from build123d import *

# Parameters (mm, degrees)
BOSS_EXTRUDE1_DEPTH      = 15.494
BOSS_EXTRUDE1_DEPTH_BACK = 15.494
SKETCH1_R                = 9.7409
SKETCH1_R_2              = 1.016
CHAMFER2_SIZE            = 4.7625
CHAMFER2_SIZE2           = 2.749630657
CHAMFER3_SIZE            = 4.7625
CHAMFER3_SIZE2           = 2.749630657


with BuildPart() as part:
    # Sketch1 → Boss-Extrude1 (new, two sides: drawn at the far end of the back side and taken through both)
    with BuildSketch(Plane.XY.offset(-BOSS_EXTRUDE1_DEPTH_BACK)):
        Circle(SKETCH1_R)
        Circle(SKETCH1_R_2, mode=Mode.SUBTRACT)
    extrude(amount=BOSS_EXTRUDE1_DEPTH + BOSS_EXTRUDE1_DEPTH_BACK)

    # Chamfer2
    chamfer2_edges = [part.edges().sort_by_distance(p)[0] for p in [
        (-9.7409, 0, -15.494),
    ]]
    chamfer2_side = [part.faces().sort_by_distance(p)[0] for p in [
        (-9.7409, 0, -7.747),
    ]]
    chamfer(chamfer2_edges, length=CHAMFER2_SIZE, length2=CHAMFER2_SIZE2, reference=chamfer2_side[0])

    # Chamfer3
    chamfer3_edges = [part.edges().sort_by_distance(p)[0] for p in [
        (-9.7409, 0, 15.494),
    ]]
    chamfer3_side = [part.faces().sort_by_distance(p)[0] for p in [
        (-9.7409, 0, 2.38125),
    ]]
    chamfer(chamfer3_edges, length=CHAMFER3_SIZE, length2=CHAMFER3_SIZE2, reference=chamfer3_side[0])


solid = part.part
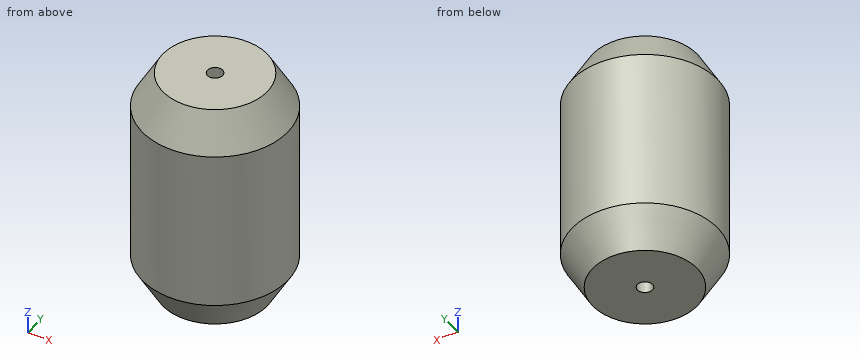
Could you check a few things on this model? Use its own coordinates, in mm. Give positions to 0.01 mm unless a question says otherwise; leave off trailing zeros. Write each loop counter-clockwise with the first axis right and the second up, starting at its lowest first coordinate (ties: lowest second). Pieces come first, ordered by that corner, then holes. Notation, with made-up numbers: (49.5, -8) -> (106.5, -8) arc R19 ccw to (106.5, 29) -> close; hole circle Ø11 at (31.25, -36.75). An arc over 180 degrees is marked (long way). Answer as a JSON object with one key per item and string values.
Q1. Suppose I cut it at D-D on z = 11.5. Write out the boundary of the cut face in (x, y), then the cut area to 3 significant figures.
Taken from the geometry:
{"outline": "circle Ø18.59 at (0, 0); hole circle Ø2.03 at (0, 0)", "area": "268 mm²"}
Q2. Suppose I cut it at A-A on x = 0. Write out the boundary of the cut face in (y, z), then the cut area to 3 significant figures.
Taken from the geometry:
{"outline": "(-9.74, -10.73) -> (-6.99, -15.49) -> (-1.02, -15.49) -> (-1.02, 15.49) -> (-6.99, 15.49) -> (-9.74, 10.73) -> close; (1.02, -15.49) -> (6.99, -15.49) -> (9.74, -10.73) -> (9.74, 10.73) -> (6.99, 15.49) -> (1.02, 15.49) -> close", "area": "515 mm²"}
Q3. Please list where these lines run through material, in increasing order: L1, parallel to Y at x = 0, z = -8; L2, parallel to X at y = -0.75, z = 2.5; L3, parallel to Y at x = -1.75, z = 8.
Taken from the geometry:
{"L1": "y = -9.74 to -1.02, 1.02 to 9.74", "L2": "x = -9.71 to -0.69, 0.69 to 9.71", "L3": "y = -9.58 to 9.58"}
Q4. Will these pins go through, and if not, where does the flat tip stop? pin 1 Ø6 at (y, z) = (-5, 7) entering from +X; pin 2 Ø1 at (y, z) = (-7.5, -9) entering from -X; pin 3 Ø1.2 at (x, y) = (0, 0) entering from -Z; pin 4 Ø2 at (x, z) = (-2, 3.5) entering from +Y.
Taken from the geometry:
{"pin 1": "stops at x = 9.53", "pin 2": "stops at x = -6.77", "pin 3": "passes through", "pin 4": "stops at y = 9.69"}
Q5. Suppose I cut it at C-C on z = -4.5. Write out the boundary of the cut face in (x, y), then the cut area to 3 significant figures.
Taken from the geometry:
{"outline": "circle Ø19.48 at (0, 0); hole circle Ø2.03 at (0, 0)", "area": "295 mm²"}
